The model under review builds one solid part; all positions refer to its coordinate system, in mm. Face numbers are marked on the shaded views. A direction names the side the tool comes from. Round coordinates to 2 decimals unless told otherwise and drop trailing zeros. Order: outer loops, then holes, each group sorted by start corner. A loop starts at its lowest first (then second) coordinate and runs counter-clockwise, first axis right, second up. Notation, with made-up numbers: (23, -9.75) -> (34, -9.75) arc R24 ccw to (34, 8.25) -> close; hole circle Ø4 at (30, 19.5). An arc over 180 degrees is marked (long way). Use a Markdown table: item, result. Add a question column.
```python
from build123d import *

# Parameters (mm, degrees)
F0_W      = 42
F0_H      = 42
F1_DEPTH  = 22
F2_W      = 21
F2_H      = 21
F3_DEPTH  = 22
F4_R      = 6
F5_DEPTH  = 22
F6_R      = 4
F7_DEPTH  = 18
F8_W      = 19
F8_H      = 19
F9_DEPTH  = 22
F10_W     = 21
F10_H     = 21
F10_R     = 6
F10_H_2   = 5
F10_W_2   = 5
F11_DEPTH = 6
F12_W     = 21
F12_H     = 21
F12_R     = 6
F12_W_2   = 5
F12_H_2   = 5
F13_DEPTH = 6
F15_R     = 6
F16_DEPTH = 15
F18_DEPTH = 34.001


with BuildPart() as f1:
    # F0 (on Top) → F1 (new body)
    with BuildSketch(Plane.XY):
        Rectangle(F0_W, F0_H)
    extrude(amount=F1_DEPTH)

    # F2 (on face) → F3 (cut, through all)
    with BuildSketch(Plane.XY.offset(22)):
        with Locations((-10.5, 10.5)):
            Rectangle(F2_W, F2_H)
    extrude(amount=-F3_DEPTH, mode=Mode.SUBTRACT)

    # F4 (on face) → F5 (cut, through all)
    with BuildSketch(Plane.XY.offset(22)):
        with Locations((10.5, -10.5)):
            Circle(F4_R)
    extrude(amount=-F5_DEPTH, mode=Mode.SUBTRACT)

    # F6 (on face) → F7 (cut)
    with BuildSketch(Plane(origin=(-21, 0, 0), x_dir=(0, -1, 0), z_dir=(-1, 0, 0))):
        with Locations((10.5, 11)):
            Circle(F6_R)
    extrude(amount=-F7_DEPTH, mode=Mode.SUBTRACT)

    # F8 (on face) → F9 (cut)
    with BuildSketch(Plane(origin=(0, 21, 0), x_dir=(-1, 0, 0), z_dir=(0, 1, 0))):
        with Locations((-10.5, 11)):
            Rectangle(F8_W, F8_H)
    extrude(amount=-F9_DEPTH, mode=Mode.SUBTRACT)

    # F10 (on face) → F11 (join)
    with BuildSketch(Plane.XY.offset(22)):
        with Locations((10.5, -10.5)):
            Rectangle(F10_W, F10_H)
        with Locations((10.5, -10.5)):
            Circle(F10_R, mode=Mode.SUBTRACT)
        with Locations((10.5, 2.5)):
            Rectangle(F10_W, F10_H_2)
        with Locations((-2.5, -10.5)):
            Rectangle(F10_W_2, F10_H)
    extrude(amount=F11_DEPTH)

    # F12 (on face) → F13 (join)
    with BuildSketch(Plane(origin=(0, 0, 0), x_dir=(1, 0, 0), z_dir=(0, 0, -1))):
        with Locations((10.5, 10.5)):
            Rectangle(F12_W, F12_H)
        with Locations((10.5, 10.5)):
            Circle(F12_R, mode=Mode.SUBTRACT)
        with Locations((-2.5, 10.5)):
            Rectangle(F12_W_2, F12_H)
        with Locations((10.5, -2.5)):
            Rectangle(F12_W, F12_H_2)
    extrude(amount=F13_DEPTH)

    # F15 (on offset) → F16 (cut, symmetric)
    with BuildSketch(Plane.XY.offset(11)):
        with BuildLine():
            Line((21, -21), (21, -10.5))
            ThreePointArc((21, -10.5), (17.9246212025, -17.9246212025), (10.5, -21))
            Line((10.5, -21), (21, -21))
        make_face()
        with BuildLine():
            Line((6.1503787975, -21), (10.5, -21))
            ThreePointArc((10.5, -21), (6.4818239602, -20.2007350914), (3.0753787975, -17.9246212025))
            Line((3.0753787975, -17.9246212025), (6.1503787975, -21))
        make_face()
        with BuildLine():
            ThreePointArc((17.9246212025, -3.0753787975), (20.2007350914, -6.4818239602), (21, -10.5))
            Line((21, -10.5), (21, -6.1503787975))
            Line((21, -6.1503787975), (17.9246212025, -3.0753787975))
        make_face()
        with BuildLine():
            ThreePointArc((10.5, -21), (17.9246212025, -17.9246212025), (21, -10.5))
            ThreePointArc((21, -10.5), (20.2007350914, -6.4818239602), (17.9246212025, -3.0753787975))
            ThreePointArc((17.9246212025, -3.0753787975), (3.0753787975, -3.0753787975), (3.0753787975, -17.9246212025))
            ThreePointArc((3.0753787975, -17.9246212025), (6.4818239602, -20.2007350914), (10.5, -21))
        make_face()
        with Locations((10.5, -10.5)):
            Circle(F15_R, mode=Mode.SUBTRACT)
    extrude(amount=F16_DEPTH, both=True, mode=Mode.SUBTRACT)

    # F17 (on face) → F18 (cut, through all)
    with BuildSketch(Plane.XY.offset(28)):
        with BuildLine():
            Line((21, -21), (21, -10.5))
            ThreePointArc((21, -10.5), (17.9246212025, -17.9246212025), (10.5, -21))
            Line((10.5, -21), (21, -21))
        make_face()
    extrude(amount=-F18_DEPTH, mode=Mode.SUBTRACT)


solid = f1.part
```
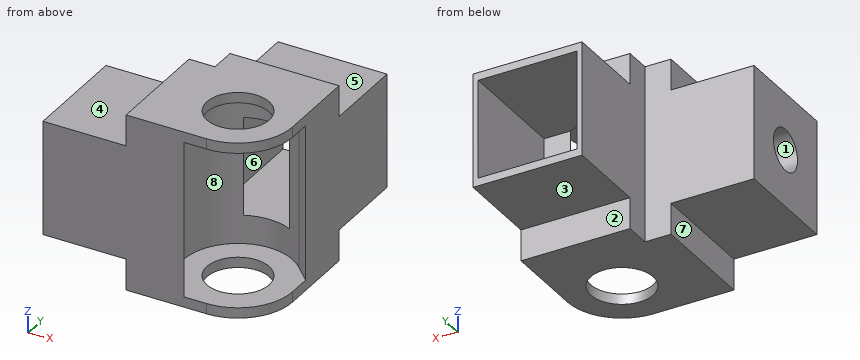
Q1. Draft analysis for pull direction Y (two halves, no side actions). For the marked faces 1, 2 and 3, state which applies: released by +Y, released by -Y, zero draft, split by the parting line, or undercut.
Q2. For the marked faces 4, 5, 6, 7 and 8, list the 3-axis set-ups (+Z, -Z, +X, -X, +Y, -Y) from which the entire face can be reached by the end or side of a thin tool; tool diameter is ignored.
Q3. To check wall thickness, follow line 1 along Z through (x, y) = (2, -11.5); line 2 along X through (y, z) = (11, 18); line 3 along Z through (x, y) = (14.5, 18). State the ranges of each line that lie inside material, in increasing order.
Q4. Add section B-B, the plane y = 17.5. Give the boundary of the cut face in (x, z), then the cut area to 3 significant figures.
Q5. Add section C-C, the plane x = -14. Give the boundary of the cut face in (y, z), then the cut area to 3 significant figures.
Q6. Add section A-A, the plane z = 11. Give the boundary of the cut face in (x, y).
Q7. For pin 1 (5 mm diameter, centred on x = 8.5, y = 11.5, fed in from +Z); pin 2 (9.5 mm diameter, centred on y = 6, z = 10, fed in from -X); pin 3 (8 mm diameter, centred on x = 9, y = 9.5, fed in from -Z), all flat-tipped, find the tip position at first contact; note any pin that passes through.
Return value:
| question | item | result |
|---|---|---|
| 1 | face 1 | undercut |
| 1 | face 2 | released by +Y |
| 1 | face 3 | zero draft |
| 2 | face 4 | +Z, -X, +Y, -Y |
| 2 | face 5 | +Z, +X, -X, +Y |
| 2 | face 6 | +Y |
| 2 | face 7 | -Z, -X, +Y, -Y |
| 2 | face 8 | none |
| 3 | line 1 | -6 to -4, 26 to 28 |
| 3 | line 2 | 0 to 1, 20 to 21 |
| 3 | line 3 | 0 to 1.5, 20.5 to 22 |
| 4 | outline | (0, 0) -> (21, 0) -> (21, 22) -> (0, 22) -> close; hole (1, 1.5) -> (20, 1.5) -> (20, 20.5) -> (1, 20.5) -> close |
| 4 | area | 101 mm² |
| 5 | outline | (-21, 0) -> (0, 0) -> (0, 22) -> (-21, 22) -> close; hole circle Ø8 at (-10.5, 11) |
| 5 | area | 412 mm² |
| 6 | outline | (-21, -21) -> (6.15, -21) -> (3.08, -17.92) arc R10.5 cw to (6.03, -1) -> (1, -1) -> (1, 21) -> (0, 21) -> (0, 0) -> (-21, 0) -> (-21, -6.5) -> (-3, -6.5) -> (-3, -14.5) -> (-21, -14.5) -> close; (14.97, -1) arc R10.5 cw to (17.92, -3.08) -> (21, -6.15) -> (21, 21) -> (20, 21) -> (20, -1) -> close |
| 7 | pin 1 | z = 22 |
| 7 | pin 2 | x = 0 |
| 7 | pin 3 | z = 0 |
